```python
from build123d import *

# Parameters (mm, degrees)
F1_DEPTH = 60


with BuildPart() as f1:
    # F0 (on Top) → F1 (new body)
    with BuildSketch(Plane.XY):
        Polygon((-0.338009, -39.998572), (34.470775, -20.29201), (34.808784, 19.706562), (0.338009, 39.998572), (-34.470775, 20.29201), (-34.808784, -19.706562), align=None)
    extrude(amount=F1_DEPTH)

    # F2 (on Right) → F3 (revolve)
    with BuildSketch(Plane.YZ):
        Polygon((20, 0), (0, 0), (0, -50), align=None)
    revolve(axis=Axis((0, 0, -25), (0, 0, -1)))


solid = f1.part
```
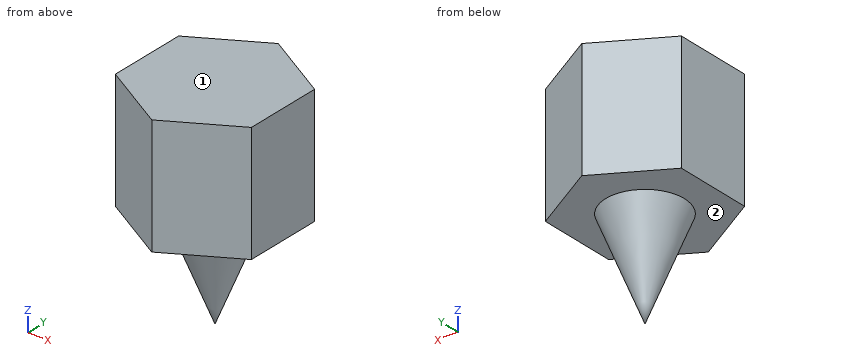
The listing builds one solid part. Answer for the finished solid, in the listing's coordinates (mm). Face numbers are marked on the shaded views. A direction names the side the tool comes from. Give positions to 0.01 mm unless a question says otherwise; leave off trailing zeros. Order: outer loops, then holes, each group sorted by start corner. A loop starts at its lowest first (then second) coordinate and runs counter-clockwise, first axis right, second up. Notation, with made-up numbers: (28, 80) -> (36, 80) arc R13 ccw to (36, 101) -> close; hole circle Ø1 at (5.25, 44.5). An arc over 180 degrees is marked (long way). Answer as CSV lines item,"result". Start each with the question number.
Q1. Given pin 1 (10 mm diameter, centred on y = -18.5, z = -21.5, fed in from -X); pin 2 (6 mm diameter, centred on x = 25.5, y = -2, fed in from -Z); pin 3 (2 mm diameter, centred on x = 13.5, z = 46.5, fed in from +Y); pin 4 (8 mm diameter, centred on y = -6.5, z = -21, fed in from +X), each flat-ended and moving along its own axis, determine where each tip first touches the part or whether it passes through.
Q2. A cutting plane is placed at C-C (z = -41). Determine the outline of the cut face in (x, y).
Q3. Which of the six approach directions +Z, -Z, +X, -X, +Y, -Y give full straight-line access (tool end or side, diameter ignored) to the marked faces 1 and 2?
Q4. Find the intervals of material crossed by L1, parallel to Z at x = 21.5, y = -19.5; L2, parallel to Z at x = -2, y = -2; L3, parallel to X at y = -15, z = 48, in increasing order.
Q5. A cutting plane is placed at A-A (z = 38). Determine the outline of the cut face in (x, y).
Q6. A cutting plane is placed at B-B (y = 23). Determine the outline of the cut face in (x, z).
Results found:
1,pin 1,"through"
1,pin 2,"z = 0"
1,pin 3,"y = 32.84"
1,pin 4,"x = 12.21"
2,outline,"circle Ø7.2 at (0, 0)"
3,face 1,"+Z, +X, -X, +Y, -Y"
3,face 2,"-Z"
4,L1,"0 to 60"
4,L2,"-42.93 to 60"
4,L3,"-34.77 to 34.52"
5,outline,"(-34.81, -19.71) -> (-0.34, -40) -> (34.47, -20.29) -> (34.81, 19.71) -> (0.34, 40) -> (-34.47, 20.29) -> close"
6,outline,"(-29.69, 0) -> (29.21, 0) -> (29.21, 60) -> (-29.69, 60) -> close"
